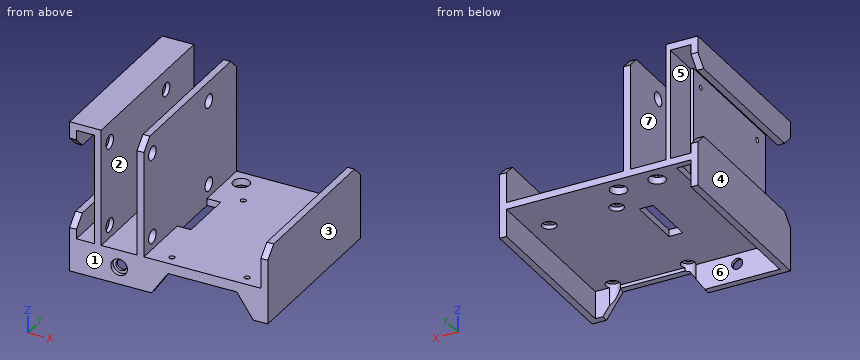
from build123d import *

# Parameters (mm, degrees)
SKETCH_R             = 4
PAD_DEPTH            = 125
SKETCH022_W          = 134
SKETCH022_H          = 125
POCKET_DEPTH         = 20
SKETCH023_R          = 6
POCKET006_DEPTH      = 3
SKETCH015_R          = 1.75
POCKET007_DEPTH      = 6
SKETCH036_R          = 5
POCKET008_DEPTH      = 3
POCKET008_DEPTH_BACK = 100
SKETCH018_R          = 2
POCKET009_DEPTH      = 25.001
SKETCH037_R          = 5
POCKET010_DEPTH      = 3
POCKET010_DEPTH_BACK = 100
SKETCH026_R          = 6
SKETCH026_W          = 10
SKETCH026_H          = 40
SKETCH026_W_2        = 13
SKETCH026_H_2        = 22.5
POCKET011_DEPTH      = 25.001
SKETCH035_W          = 80
SKETCH035_H          = 27.5
POCKET012_DEPTH      = 2
CHAMFER_SIZE         = 8


with BuildPart() as part:
    # Sketch → Pad (new body)
    with BuildSketch(Plane.XZ):
        Polygon((144, 0), (144, 55), (139, 55), (139, 25), (54, 25), (54, 110), (49, 110), (49, 25), (23, 25), (23, 110), (0, 110), (0, 90), (5, 90), (5, 105), (18, 105), (18, 25), (5, 25), (5, 40), (0, 40), (0, 0), (59.5, 0), (71.5, 17.5), (121.5, 17.5), (133.5, 0), align=None)
        with Locations((36, 12.5)):
            Circle(SKETCH_R, mode=Mode.SUBTRACT)
    extrude(amount=PAD_DEPTH)

    # Sketch022 (on Face20 of Pad) → Pocket (cut)
    with BuildSketch(Plane(origin=(0, 0, 0), x_dir=(1, 0, 0), z_dir=(0, 0, -1))):
        with Locations((72, 57.5)):
            Rectangle(SKETCH022_W, SKETCH022_H)
    extrude(amount=-POCKET_DEPTH, mode=Mode.SUBTRACT)

    # Sketch023 (on Face5 of Pocket) → Pocket006 (cut)
    with BuildSketch(Plane.XZ.offset(125)):
        with Locations((36, 12.5)):
            Circle(SKETCH023_R)
    extrude(amount=-POCKET006_DEPTH, mode=Mode.SUBTRACT)

    # Sketch015 (on Face17 of Pocket006) → Pocket007 (cut)
    with BuildSketch(Plane(origin=(18, 0, 0), x_dir=(0, 0, -1), z_dir=(-1, 0, 0))):
        with Locations((-95.675, 113.6)):
            Circle(SKETCH015_R)
        with Locations((-34.325, 113.6)):
            Circle(SKETCH015_R)
        with Locations((-34.325, 37.45)):
            Circle(SKETCH015_R)
        with Locations((-95.675, 37.45)):
            Circle(SKETCH015_R)
    extrude(amount=-POCKET007_DEPTH, mode=Mode.SUBTRACT)

    # Sketch036 (on Face23 of Pocket007) → Pocket008 (cut, two sides)
    with BuildSketch(Plane(origin=(23, 0, 0), x_dir=(0, 0, 1), z_dir=(1, 0, 0))) as pocket008_sk:
        with Locations((95.675, 113.6)):
            Circle(SKETCH036_R)
        with Locations((34.325, 113.6)):
            Circle(SKETCH036_R)
        with Locations((34.325, 37.45)):
            Circle(SKETCH036_R)
        with Locations((95.675, 37.45)):
            Circle(SKETCH036_R)
    extrude(amount=-POCKET008_DEPTH, mode=Mode.SUBTRACT)
    extrude(pocket008_sk.sketch, amount=POCKET008_DEPTH_BACK, mode=Mode.SUBTRACT)

    # Sketch018 (on Face28 of Pocket008) → Pocket009 (cut, through all)
    with BuildSketch(Plane(origin=(0, 0, 25), x_dir=(-1, 0, 0), z_dir=(0, 0, 1))):
        with Locations((-124.69, 117)):
            Circle(SKETCH018_R)
        with Locations((-70, 117)):
            Circle(SKETCH018_R)
        with Locations((-124.69, 31.14)):
            Circle(SKETCH018_R)
        with Locations((-75.71, 31.14)):
            Circle(SKETCH018_R)
    extrude(amount=-POCKET009_DEPTH, mode=Mode.SUBTRACT)

    # Sketch037 (on Face10 of Pocket009) → Pocket010 (cut, two sides)
    with BuildSketch(Plane(origin=(0, 0, 20), x_dir=(1, 0, 0), z_dir=(0, 0, -1))) as pocket010_sk:
        with Locations((70, 117)):
            Circle(SKETCH037_R)
        with Locations((124.69, 117)):
            Circle(SKETCH037_R)
        with Locations((75.71, 31.14)):
            Circle(SKETCH037_R)
        with Locations((124.69, 31.14)):
            Circle(SKETCH037_R)
    extrude(amount=-POCKET010_DEPTH, mode=Mode.SUBTRACT)
    extrude(pocket010_sk.sketch, amount=POCKET010_DEPTH_BACK, mode=Mode.SUBTRACT)

    # Sketch026 (on Face28 of Pocket010) → Pocket011 (cut, through all)
    with BuildSketch(Plane(origin=(0, 0, 25), x_dir=(-1, 0, 0), z_dir=(0, 0, 1))):
        with Locations((-36, 12)):
            Circle(SKETCH026_R)
        with Locations((-64, 12)):
            Circle(SKETCH026_R)
        with Locations((-59, 60)):
            Rectangle(SKETCH026_W, SKETCH026_H)
        with Locations((-11.5, 16.25)):
            Rectangle(SKETCH026_W_2, SKETCH026_H_2)
    extrude(amount=-POCKET011_DEPTH, mode=Mode.SUBTRACT)

    # Sketch035 (on Face17 of Pocket011) → Pocket012 (cut)
    with BuildSketch(Plane(origin=(18, 0, 0), x_dir=(0, 0, -1), z_dir=(-1, 0, 0))):
        with Locations((-65, 13.75)):
            Rectangle(SKETCH035_W, SKETCH035_H)
    extrude(amount=-POCKET012_DEPTH, mode=Mode.SUBTRACT)

    # Chamfer
    chamfer_edges = [part.edges().sort_by_distance(p)[0] for p in [
        (51.5, -125, 110),
        (2.5, -125, 90),
        (2.5, -125, 40),
        (141.5, -125, 55),
        (141.5, 0, 55),
        (2.5, 0, 40),
        (2.5, 0, 90),
        (51.5, 0, 110),
    ]]
    chamfer(chamfer_edges, length=CHAMFER_SIZE)


solid = part.part
For this review, take the finished solid that the model builds, in its own axes (mm). Face numbers are marked on the shaded views. A direction names the side the tool comes from. Round coordinates to 2 decimals unless told otherwise and drop trailing zeros. Order: outer loops, then holes, each group sorted by start corner. A loop starts at its lowest first (then second) coordinate and runs counter-clockwise, first axis right, second up. Notation, with made-up numbers: M 47,58 L 85,58 A16 cw 85,67 Z; hole C 88,-2 d10. An arc over 180 degrees is marked long. Use a Markdown table: item, result. Add a question column.
Item 1: Mouldability with a two-part tool opening along X and no side actions: class the marked faces 1, 2, 3 and 4 as released by +X, released by -X, zero draft, split by the parting line, or undercut.
Item 2: Add section C-C, the plane z = 71.5. Give the boundary of the cut face in (x, y).
Item 3: Add section B-B, the plane y = -12. State how many separate pieces and enclosed holes the cut face has, then the cut area to 4 significant figures.
Item 4: Tool access review of the marked faces 5, 6 and 7: name each direction out of +Z, -Z, +X, -X, +Y, -Y from which nothing blocks a thin tool from reaching the whole face with its end or side.
Item 5: Add section D-D, the plane y = -49. Give the boundary of the cut face in (x, z), then the cut area to 3 significant figures.
Item 6: To check wall thickness, follow line 1 along X through (y, z) = (-54.5, 41.5); line 2 along X through (y, z) = (-79, 93.5); line 3 along X through (y, z) = (-36.5, 33). State the ranges of each line that lie inside material, in increasing order.
Item 7: Insertion check: pin 1 (1.5 mm diameter, centred on x = 58.5, z = 23, fed in from +Y); pin 2 (6.5 mm diameter, centred on x = 75.71, y = -31.14, fed in from -Z); pin 3 (14 mm diameter, centred on y = -18.5, z = 61.5, fed in from -X); pin 4 (6 mm diameter, centred on y = -113.6, z = 95.675, fed in from +X). Each pin has a flat end and moves straight along its axis. Give the tip position at first contact, or say it passes through.
Item 8: Add section A-A, the plane z = 43. Give the boundary of the cut face in (x, y), then the cut area to 3 significant figures.
Geometry results:
| question | item | result |
|---|---|---|
| 1 | face 1 | zero draft |
| 1 | face 2 | undercut |
| 1 | face 3 | released by +X |
| 1 | face 4 | released by -X |
| 2 | outline | M 18,-125 L 23,-125 L 23,0 L 20,0 L 20,-27.5 L 18,-27.5 Z; M 49,-125 L 54,-125 L 54,0 L 49,0 Z |
| 3 | separate pieces | 4 |
| 3 | enclosed holes | 0 |
| 3 | area | 1,815 mm² |
| 4 | face 5 | +Y |
| 4 | face 6 | -Z, +Y |
| 4 | face 7 | +Z, +Y, -Y |
| 5 | outline | M 0,0 L 5,0 L 5,20 L 54,20 L 54,110 L 49,110 L 49,25 L 23,25 L 23,110 L 0,110 L 0,90 L 5,90 L 5,105 L 18,105 L 18,25 L 5,25 L 5,40 L 0,40 Z; M 64,20 L 139,20 L 139,0 L 144,0 L 144,55 L 139,55 L 139,25 L 64,25 Z |
| 5 | area | 2,110 mm² |
| 6 | line 1 | x = 18 to 23, 49 to 54, 139 to 144 |
| 6 | line 2 | x = 0 to 5, 18 to 23, 49 to 54 |
| 6 | line 3 | x = 0 to 5, 139 to 144 |
| 7 | pin 1 | stops at y = 0 |
| 7 | pin 2 | stops at z = 23 |
| 7 | pin 3 | stops at x = 20 |
| 7 | pin 4 | stops at x = 20 |
| 8 | outline | M 18,-125 L 23,-125 L 23,0 L 20,0 L 20,-27.5 L 18,-27.5 Z; M 49,-125 L 54,-125 L 54,0 L 49,0 Z; M 139,-125 L 144,-125 L 144,0 L 139,0 Z |
| 8 | area | 1,820 mm² |
